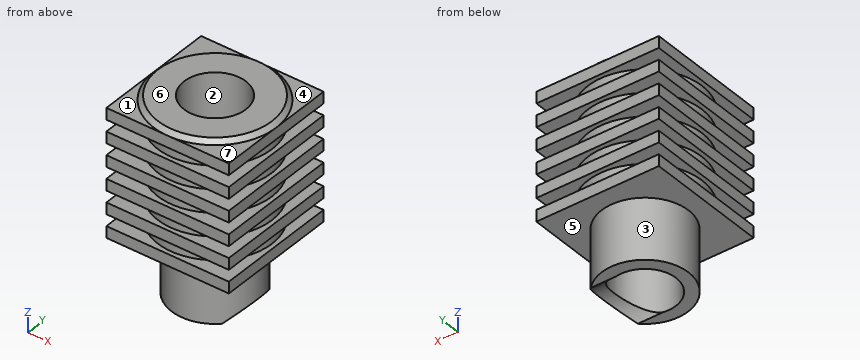
```python
from build123d import *

# Parameters (mm, degrees)
F2_W     = 35.9156
F2_H     = 35.9156
F3_DEPTH = 56.3128
F5_DEPTH = 13.7000001


with BuildPart() as f1:
    # F0 (on Front) → F1 (revolve)
    with BuildSketch(Plane.XZ):
        Polygon((12.8905, 56.3118), (12.8905, 55.0418), (17.9705, 55.0418), (16.7005, 56.3118), align=None)
        Polygon((17.9705, 55.0418), (12.8905, 55.0418), (12.8905, 17.7884666667), (17.9705, 17.7884666667), (50.8, 17.7884666667), (50.8, 21.1751333333), (16.7005, 21.1751333333), (16.7005, 24.5618), (50.8, 24.5618), (50.8, 27.9484666667), (16.7005, 27.9484666667), (16.7005, 31.3351333333), (50.8, 31.3351333333), (50.8, 34.7218), (16.7005, 34.7218), (16.7005, 38.1084666667), (50.8, 38.1084666667), (50.8, 41.4951333333), (16.7005, 41.4951333333), (16.7005, 44.8818), (50.8, 44.8818), (50.8, 48.2684666667), (16.7005, 48.2684666667), (16.7005, 51.6551333333), (50.8, 51.6551333333), (50.8, 55.0418), align=None)
        Polygon((12.8905, 17.7884666667), (12.8905, 55.0418), (12.8905, 56.3118), (9.0805, 56.3118), (9.0805, 0), (12.7, 0), (12.7, 17.7884666667), align=None)
    revolve(axis=Axis((0, 0, 27.5209), (0, 0, 1)))

    # F2 (on face) → F3 (cut, through all)
    with BuildSketch(Plane.XY.offset(56.3118)):
        with BuildLine():
            ThreePointArc((50.8, 0), (35.9210245024, 35.9210244661), (5.14e-08, 50.8))
            ThreePointArc((5.14e-08, 50.8), (-35.9210245011, 35.9210244675), (-50.8, -9.89e-08))
            ThreePointArc((-50.8, -9.89e-08), (-35.9210244493, -35.9210245192), (0, -50.8))
            ThreePointArc((0, -50.8), (35.9210244843, -35.9210244843), (50.8, 0))
        make_face()
        Rectangle(F2_W, F2_H, mode=Mode.SUBTRACT)
    extrude(amount=-F3_DEPTH, mode=Mode.SUBTRACT)

    # F4 (on Right) → F5 (cut, up to face)
    with BuildSketch(Plane.YZ):
        with BuildLine():
            ThreePointArc((-8.9408, 0), (-4.8805494132, -20.7288154777), (12.6937813793, -9.0107813793))
            ThreePointArc((12.6937813793, -9.0107813793), (11.7180340984, -4.1302319661), (8.9408, 0))
            Line((8.9408, 0), (-8.9408, 0))
        make_face()
        with BuildLine():
            Line((-8.9408, 0), (8.9408, 0))
            ThreePointArc((8.9408, 0), (0, 3.683), (-8.9408, 0))
        make_face()
    extrude(amount=F5_DEPTH, mode=Mode.SUBTRACT)


solid = f1.part
```
Work out the finished part from the listing and answer in its coordinate system (mm). Face numbers are marked on the shaded views. A direction names the side the tool comes from. Coordinates: 2 decimals unless noted, no trailing zeros. Order: outer loops, then holes, each group sorted by start corner. A loop starts at its lowest first (then second) coordinate and runs counter-clockwise, first axis right, second up. Notation, with made-up numbers: (-7.5, 72.5) - (25.5, 72.5) arc R22 cw to (25.5, 109.5) - close; hole circle Ø8 at (39.25, 86). An arc over 180 degrees is marked (long way). Answer as a JSON object with one key per item and string values.
1. The mould has two halves that part along Y. Classify the marked faces 1, 2 and 3: +Y half, -Y half, draft (parallel to the pull), parting line (faces both ways), or undercut.
Output values:
{"face 1": "draft", "face 2": "undercut", "face 3": "parting line"}
2. Consider line 1 (Z direction, x = 12.5, y = 13.5); line 2 (Y direction, x = 0, z = 25.5); line 3 (X direction, y = 0, z = 17). Determine where each line is inside the solid, lowest interval first.
Output values:
{"line 1": "z = 17.79 to 21.18, 24.56 to 27.95, 31.34 to 34.72, 38.11 to 41.5, 44.88 to 48.27, 51.66 to 55.04", "line 2": "y = -17.96 to -9.08, 9.08 to 17.96", "line 3": "x = -12.7 to -9.08, 9.08 to 12.7"}
3. Each of these flat-tipped pins is pushed along its axis until it touches: P1, Ø11, axis at x = 0, y = 0, coming from the -Z side; P2, Ø12, axis at x = 14, y = -11.5, coming from the -Z side. Where does it stop, or does it pass through?
Output values:
{"P1": "passes through", "P2": "stops at z = 0"}
4. Find section A-A on z = 5.5. Determine the outline of the cut face in (x, y), plus the area to 3 significant figures.
Output values:
{"outline": "circle Ø25.4 at (0, 0); hole circle Ø18.16 at (0, 0)", "area": "248 mm²"}
5. A tool of negligible diameter and unlimited length cuts with its end or side. For the marked faces 4, 5, 6 and 7, from which of +Z, -Z, +X, -X, +Y, -Y can it reach the whole face along a straight path? Write none if from no direction.
Output values:
{"face 4": "+Z, +X, +Y", "face 5": "-Z", "face 6": "+Z, +X, -X, +Y, -Y", "face 7": "+Z, +X, -Y"}
